Source: CAD feature listing. Evaluate the final solid. Frame: model axes, mm. A direction names the side the tool comes from. Round coordinates to 2 decimals unless told otherwise and drop trailing zeros. Loops run counter-clockwise (first coordinate to the right, second up) from the corner with the lowest first, then second, coordinate; pieces in that order, holes last.
(1) First-contact query: pin 1 Ø4 at (y, z) = (4.5, 13.5) entering from +X; pin 2 Ø13.5 at (x, y) = (10.5, -19.5) entering from +Z (3 decimals); pin 3 Ø1 at (x, z) = (35, 9.5) entering from +Y; pin 4 Ø4 at (x, y) = (-15, -30.5) entering from -Z. Flat tips, straight axial feed; report the tip coordinate or a pass-through.
(2) Section A-A, the plane z = 46. Return the cut outline in (x, y).
(3) Material intervals for probe 1 along X at (y, z) = (0, 2); probe 2 along Z at (x, y) = (40.5, -22) (3 decimals); probe 3 along Z at (x, y) = (-11, -30) (3 decimals), sorted ascending.
(4) Section B-B, the plane x = 1. Return the cut outline in (y, z) (3 decimals).
(5) Mould query, pull axis Y, two halves, no side actions, for faces 1 (the cylindrical face through (53.046, -2.399, 67.033)), 2 (the cylindrical face through (-39.264, -17.917, 1.61)), 3 (the cylindrical face through (35.864, -32.158, 71.315)), 4 (the cylindrical face through (53.133, -2.248, 54.017)). Classes: pulls with the +Y half, pulls with the -Y half, needs draft (parallel to the pull), parting line crosses it, or undercut.
(6) Set-up query: faces 5 (the flat face through (45.67, -12.04, 37.71)), 6 (the cylindrical face through (41.353, -22.653, 28.617)), 7 (the flat face through (39.325, -26.165, 35.089)), 8 (the cylindrical face through (17.91, 5.36, 1.57)), 9 (the flat face through (11.811, -33.958, 1.565)). Return all of +Z, -Z, +X, -X, +Y, -Y with unobstructed straight access to the full face (end or side cutting, diameter ignored); none if empty.
```python
from build123d import *

# Parameters (mm, degrees)
SKETCH3_R           = 5.2705
BOSS_EXTRUDE1_DEPTH = 3.175
BOSS_EXTRUDE2_DEPTH = 70.05
FILLET1_R           = 12.7
FILLET3_R           = 25.4
SKETCH5_R           = 3.96875
CUT_EXTRUDE1_DEPTH  = 6.35
FILLET4_R           = 6.35


with BuildPart() as part:
    # Sketch3 → Boss-Extrude1 (new body)
    with BuildSketch(Plane.XY):
        with BuildLine():
            Line((-31.875, 1.314467847), (-31.875, 2.123689729))
            Line((-31.875, 2.123689729), (-44.309751158, -19.413931056))
            Line((-44.309751158, -19.413931056), (-16.813444588, -35.288931056))
            Line((-16.813444588, -35.288931056), (33.603324087, -32.943986013))
            Line((33.603324087, -32.943986013), (36.352954744, -34.531486013))
            Line((36.352954744, -34.531486013), (60.833371586, 7.869839748))
            Line((60.833371586, 7.869839748), (58.083740929, 9.457339748))
            Line((58.083740929, 9.457339748), (23.441464566, 7.84608547))
            ThreePointArc((23.441464566, 7.84608547), (28.824079828, 6.169187612), (31.875, 1.428257367))
            ThreePointArc((31.875, 1.428257367), (32.028589915, 0.519857326), (32.08, -0.4))
            ThreePointArc((32.08, -0.4), (32.028589915, -1.319857326), (31.875, -2.228257367))
            Line((31.875, -2.228257367), (31.875, -6.284053394))
            ThreePointArc((31.875, -6.284053394), (21.132205448, -10.12115273), (9.948783703, -12.371051434))
            ThreePointArc((9.948783703, -12.371051434), (0.015428746, -15.957499724), (-9.919275826, -12.374791656))
            ThreePointArc((-9.919275826, -12.374791656), (-21.117875037, -10.125129582), (-31.875, -6.284053394))
            Line((-31.875, -6.284053394), (-31.875, -2.114467847))
            ThreePointArc((-31.875, -2.114467847), (-32.055, -0.4), (-31.875, 1.314467847))
        make_face()
        with BuildLine():
            ThreePointArc((15.57, -0.4), (14.094750174, -7.012566542), (9.948783703, -12.371051434))
            ThreePointArc((9.948783703, -12.371051434), (21.132205448, -10.12115273), (31.875, -6.284053394))
            Line((31.875, -6.284053394), (31.875, -2.228257367))
            ThreePointArc((31.875, -2.228257367), (22.905142674, -8.603589915), (15.57, -0.4))
        make_face()
        with BuildLine():
            ThreePointArc((23.441464566, 7.84608547), (17.853772739, 5.299953508), (15.57, -0.4))
            ThreePointArc((15.57, -0.4), (22.905142674, -8.603589915), (31.875, -2.228257367))
            Line((31.875, -2.228257367), (31.875, 1.428257367))
            ThreePointArc((31.875, 1.428257367), (28.824079828, 6.169187612), (23.441464566, 7.84608547))
        make_face()
        with Locations((23.825, -0.4)):
            Circle(SKETCH3_R, mode=Mode.SUBTRACT)
        with BuildLine():
            ThreePointArc((-9.919275826, -12.374791656), (-14.068505089, -7.015217451), (-15.545, -0.4))
            ThreePointArc((-15.545, -0.4), (-22.938054526, -8.609876674), (-31.875, -2.114467847))
            Line((-31.875, -2.114467847), (-31.875, -6.284053394))
            ThreePointArc((-31.875, -6.284053394), (-21.117875037, -10.125129582), (-9.919275826, -12.374791656))
        make_face()
        with BuildLine():
            ThreePointArc((-15.545, -0.4), (-21.663448783, 7.573717696), (-30.949039708, 3.7275))
            ThreePointArc((-30.949039708, 3.7275), (-31.507044005, 2.557447835), (-31.875, 1.314467847))
            Line((-31.875, 1.314467847), (-31.875, -2.114467847))
            ThreePointArc((-31.875, -2.114467847), (-22.938054526, -8.609876674), (-15.545, -0.4))
        make_face()
        with Locations((-23.8, -0.4)):
            Circle(SKETCH3_R, mode=Mode.SUBTRACT)
        with BuildLine():
            Line((31.875, 1.428257367), (31.875, -2.228257367))
            ThreePointArc((31.875, -2.228257367), (32.028589915, -1.319857326), (32.08, -0.4))
            ThreePointArc((32.08, -0.4), (32.028589915, 0.519857326), (31.875, 1.428257367))
        make_face()
        with BuildLine():
            Line((-31.875, -2.114467847), (-31.875, 1.314467847))
            ThreePointArc((-31.875, 1.314467847), (-32.055, -0.4), (-31.875, -2.114467847))
        make_face()
        with BuildLine():
            ThreePointArc((-31.875, 1.314467847), (-31.507044005, 2.557447835), (-30.949039708, 3.7275))
            Line((-30.949039708, 3.7275), (-31.875, 2.123689729))
            Line((-31.875, 2.123689729), (-31.875, 1.314467847))
        make_face()
    extrude(amount=BOSS_EXTRUDE1_DEPTH)

    # Sketch4 → Boss-Extrude2 (add)
    with BuildSketch(Plane.XY.offset(3.175)):
        Polygon((60.833371586, 7.869839748), (36.352954744, -34.531486013), (33.603324087, -32.943986013), (58.083740929, 9.457339748), align=None)
    extrude(amount=BOSS_EXTRUDE2_DEPTH)

    # Fillet1
    fillet1_edges = [part.edges().sort_by_distance(p)[0] for p in [
        (-44.309751158, -19.413931056, 1.5875),
    ]]
    fillet(fillet1_edges, radius=FILLET1_R)

    # Fillet3
    fillet3_edges = [part.edges().sort_by_distance(p)[0] for p in [
        (-16.813444588, -35.288931056, 1.5875),
    ]]
    fillet(fillet3_edges, radius=FILLET3_R)

    # Sketch5 → Cut-Extrude1 (cut)
    with BuildSketch(Plane(origin=(39.46765746, -22.786662659, 0), x_dir=(0, 0, 1), z_dir=(-0.866025404, 0.5, 0))):
        with Locations((63.065, 24.532166939)):
            Circle(SKETCH5_R)
        with Locations((57.985, 24.532166939)):
            Circle(SKETCH5_R)
        with BuildLine():
            ThreePointArc((60.525, 21.482679021), (59.335614932, 20.800302007), (57.985, 20.563416939))
            Line((57.985, 20.563416939), (63.065, 20.563416939))
            ThreePointArc((63.065, 20.563416939), (61.714385068, 20.800302007), (60.525, 21.482679021))
        make_face()
        with BuildLine():
            Line((63.065, 28.500916939), (57.985, 28.500916939))
            ThreePointArc((57.985, 28.500916939), (59.335614932, 28.26403187), (60.525, 27.581654857))
            ThreePointArc((60.525, 27.581654857), (61.714385068, 28.26403187), (63.065, 28.500916939))
        make_face()
        with Locations((37.665, 0.971333254)):
            Circle(SKETCH5_R)
        with Locations((32.585, 0.971333254)):
            Circle(SKETCH5_R)
        with BuildLine():
            Line((37.665, 4.940083254), (32.585, 4.940083254))
            ThreePointArc((32.585, 4.940083254), (33.935614932, 4.703198186), (35.125, 4.020821172))
            ThreePointArc((35.125, 4.020821172), (36.314385068, 4.703198186), (37.665, 4.940083254))
        make_face()
        with BuildLine():
            ThreePointArc((35.125, -2.078154664), (33.935614932, -2.760531678), (32.585, -2.997416746))
            Line((32.585, -2.997416746), (37.665, -2.997416746))
            ThreePointArc((37.665, -2.997416746), (36.314385068, -2.760531678), (35.125, -2.078154664))
        make_face()
    extrude(amount=-CUT_EXTRUDE1_DEPTH, mode=Mode.SUBTRACT)

    # Fillet4
    fillet4_edges = [part.edges().sort_by_distance(p)[0] for p in [
        (34.978139415, -33.737736013, 73.225),
        (59.458556258, 8.663589748, 73.225),
    ]]
    fillet(fillet4_edges, radius=FILLET4_R)


solid = part.part
```
Output values:
1. pin 1: stops at x = 60.04
1. pin 2: stops at z = 3.175
1. pin 3: stops at y = -29.66
1. pin 4: stops at z = 0
2. outline: (33.6, -32.94) - (36.35, -34.53) - (60.83, 7.87) - (58.08, 9.46) - close
3. probe 1: x = -33.1 to -29.06, -18.54 to -15.55, 15.58 to 18.57, 29.08 to 56.29
3. probe 2: z = 0 to 28.623, 41.627 to 73.225
3. probe 3: z = 0 to 3.175
4. outline: (-34.46, 0) - (-15.926, 0) - (-15.926, 3.175) - (-34.46, 3.175) - close
5. face 1: undercut
5. face 2: parting line crosses it
5. face 3: pulls with the -Y half
5. face 4: undercut
6. face 5: +Z, -X, +Y
6. face 6: none
6. face 7: +X, +Y
6. face 8: +Z, -Z, +Y
6. face 9: +Z, -Z, -Y
